Work out the finished part from the listing and answer in its coordinate system (mm). Face numbers are marked on the shaded views. A direction names the side the tool comes from. Round coordinates to 2 decimals unless told otherwise and drop trailing zeros. Order: outer loops, then holes, each group sorted by start corner. A loop starts at its lowest first (then second) coordinate and runs counter-clockwise, first axis right, second up. Notation, with made-up numbers: (31, 46) -> (40, 46) arc R13 ccw to (40, 53) -> close; hole circle Ø7 at (7, -9). An arc over 180 degrees is marked (long way). Use a Markdown table: item, result. Add a question column.
Item 1: A cutting plane is placed at D-D, the plane z = 23. Determine the outline of the cut face in (x, y), plus the area to 3 significant figures.
Item 2: Find the intervals of material crossed by L1, parallel to Z at x = 0, y = -13.25; L2, parallel to Z at x = 0, y = -18.35; L3, parallel to X at y = -17.5, z = -29, in increasing order. Write a range as [from, to].
Item 3: Flat-ended cylindrical pins translate along their axes: P1, Ø3, axis at x = 0.5, y = 2, coming from the -Z side; P2, Ø9.5, axis at x = 0, z = 23, coming from the +Y side; P3, Ø0.8, axis at x = 1, y = -17.5, coming from the -Z side; P4, Ø5.5, axis at x = 0, z = -7, coming from the -Y side. Find the tip coordinate at first contact, or state that the pin passes through.
Item 4: A cutting plane is placed at A-A, the plane z = -29.5. Determine the outline of the cut face in (x, y), plus the area to 3 significant figures.
Item 5: A tool of negligible diameter and unlimited length cuts with its end or side. For the marked faces 1, 2 and 3, from which of +Z, -Z, +X, -X, +Y, -Y can it reach the whole face along a straight path? Write none if from no direction.
Item 6: A cutting plane is placed at B-B, the plane z = -7. Determine the outline of the cut face in (x, y).
Item 7: For a pull along X with two mould halves and no side action, classify the marked faces 4, 5 and 6 as +X half, -X half, draft (parallel to the pull), parting line (faces both ways), or undercut.
Item 8: A cutting plane is placed at C-C, the plane y = -1.25. Determine the outline of the cut face in (x, z).
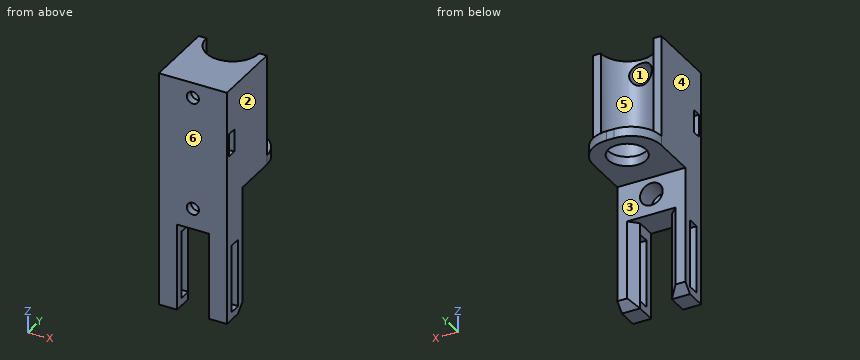
Autodesk Inventor part; units mm, degrees
ref_plane "YZ Plane" through (0, 0, 0) normal (1, 0, 0) x (0, 1, 0)
ref_plane "XZ Plane" through (0, 0, 0) normal (0, 1, 0) x (-1, 0, 0)
ref_plane "XY Plane" through (0, 0, 0) normal (0, 0, 1) x (1, 0, 0)
sketch "Sketch1" plane through (0, 0, 0) normal (0, 0, 1) x (1, 0, 0)
  circle A0 centre (0, 0) radius 7
  circle A1 centre (0, 0) radius 5
  circle A2 centre (0, 0) radius 1
  line L0 (-9, 0) -> (9, 0)
  line L1 (9, 0) -> (9, -19)
  line L2 (9, -19) -> (-9, -19)
  line L3 (-9, -19) -> (-9, 0)
  dimension "d11" = 14
  dimension "d12" = 10
  dimension "d13" = 2
  dimension "d18" = 19
  dimension "d19" = 18
extrude "Extrusion1" add sketch "Sketch1" along normal blind 27 contours L0 L1 L2 L3 A0 | A0 L0 A1 | A1 L0 A2 | A2 L0 picked at (6.2655, -0.5584) picked at (3.6182, -0.3989) picked at (-0.2952, -0.1549)
sketch "Sketch3" plane through (0, 0, 0) normal (0, 0, -1) x (-1, 0, 0)
  line L0 (9, -19) -> (9, 0)
  line L1 (-9, -19) -> (9, -19)
  line L2 (9, -19) -> (9, 8)
  line L3 (9, 8) -> (-9, 8)
  line L4 (-9, 8) -> (-9, -19)
  dimension "d22" = 27
extrude "Extrusion6" add sketch "Sketch3" along normal blind 2.5
extrude "Extrusion5" cut sketch "Sketch1" along normal blind 30 contours L0 A1 A0 | A0 L0 A1 | L0 A2 A1 | A1 L0 A2 | L0 A2 | A2 L0
extrude "Extrusion7" cut sketch "Sketch1" against normal through all contours L0 A2 A1 | A1 L0 A2 | L0 A2 | A2 L0
fillet "Fillet1" radius 8 2 edges at (-9, 8, -1.25) (9, 8, -1.25)
sketch "Sketch4" plane through (9, -19, 27) normal (1, 0, 0) x (0, 0, -1)
  line L0 (0, 0) -> (29.5, 0)
  line L1 (11.75, 3.5) -> (17.75, 3.5)
  line L2 (17.75, 3.5) -> (17.75, 1)
  line L3 (17.75, 1) -> (11.75, 1)
  line L4 (11.75, 1) -> (11.75, 3.5)
  point P0 (14.75, 0)
  point P1 (14.75, 1)
  dimension "d32" = 6
  dimension "d33" = 2.5
  dimension "d34" = 1
extrude "Extrusion8" cut sketch "Sketch4" against normal through all
sketch "Sketch5" plane through (0, 0, -2.5) normal (0, 0, -1) x (-1, 0, 0)
  line L0 (9, -19) -> (9, 0)
  line L1 (-9, -19) -> (9, -19)
  line L2 (9, -19) -> (9, -11.5)
  line L3 (9, -11.5) -> (-9, -11.5)
  line L4 (-9, -11.5) -> (-9, -19)
  dimension "d37" = 7.5
extrude "Extrusion9" add sketch "Sketch5" along normal blind 33
sketch "Sketch6" plane through (-9, -11.5, -2.5) normal (0, 1, 0) x (1, 0, 0)
  line L0 (4.8, 10) -> (13.2, 10)
  line L1 (13.2, 10) -> (13.2, 33)
  line L2 (13.2, 33) -> (4.8, 33)
  line L3 (4.8, 33) -> (4.8, 10)
  line L4 (0, 33) -> (18, 33)
  point P0 (9, -2.5)
  point P1 (9, 33)
  point P2 (9, 33)
  dimension "d45" = 23
  dimension "d47" = 0
  dimension "d69" = 8.4
extrude "Extrusion10" cut sketch "Sketch6" against normal blind 30
sketch "Sketch7" plane through (9, -19, 27) normal (1, 0, 0) x (0, 0, -1)
  line L0 (42.5, 5.35) -> (60.5, 5.35)
  line L1 (60.5, 5.35) -> (60.5, 2.15)
  line L2 (60.5, 2.15) -> (42.5, 2.15)
  line L3 (42.5, 2.15) -> (42.5, 5.35)
  line L4 (62.5, 7.5) -> (62.5, 0)
  line L5 (62.5, 7.5) -> (39.5, 7.5)
  point P0 (27, 19)
  point P1 (60.5, 3.75)
  point P2 (62.5, 3.75)
  point P3 (51.5, 5.35)
  point P4 (51, 7.5)
  point P5 (59.5, 7.5)
  dimension "d49" = 3.2
  dimension "d55" = 18
  dimension "d70" = 20
extrude "Extrusion11" cut sketch "Sketch7" against normal through all
sketch "Sketch8" plane through (-9, -11.5, -2.5) normal (0, 1, 0) x (1, 0, 0)
  circle A0 centre (9, 4.5) radius 3
  circle A1 centre (9, -25.5) radius 3
  line L0 (16, -29.5) -> (2, -29.5)
  point P0 (9, -2.5)
  dimension "d56" = 6
  dimension "d57" = 6
  dimension "d58" = 4
  dimension "d59" = 34
extrude "Extrusion12" cut sketch "Sketch8" along normal mid plane 11
sketch "Sketch9" plane through (0, -17, -7) normal (0, 1, 0) x (1, 0, 0)
  circle A0 centre (0, 0) radius 3
  circle A1 centre (0, 0) radius 1.6
  circle A2 centre (0, -30) radius 1.6
  point P0 (0, -7)
  dimension "d62" = 3.2
  dimension "d63" = 3.2
extrude "Extrusion13" cut sketch "Sketch9" against normal through all contours A1 | A2
chamfer "Chamfer2" distance 2.2 angle 45 4 edges at (4.2, -11.5, -24) (-4.2, -11.5, -24) (6.6, -11.5, -35.5) (-6.6, -11.5, -35.5)
properties part number "Solinoid holder v5"
Reported:
| question | item | result |
|---|---|---|
| 1 | outline | (-9, -19) -> (-1.6, -19) -> (-1.6, -17) -> (-3, -17) -> (-3, -6.32) arc R7 cw to (-7, 0) -> (-9, 0) -> close; (1.6, -19) -> (9, -19) -> (9, 0) -> (7, 0) arc R7 cw to (3, -6.32) -> (3, -17) -> (1.6, -17) -> close |
| 1 | area | 197 mm² |
| 2 | L1 | [-12.5, -10], [-4, 20], [26, 27] |
| 2 | L2 | [-12.5, -8.6], [-5.4, 21.4], [24.6, 27] |
| 2 | L3 | [-9, -4.2], [4.2, 9] |
| 3 | P1 | through |
| 3 | P2 | y = -5.14 |
| 3 | P3 | z = -12.5 |
| 3 | P4 | y = -19 |
| 4 | outline | (-9, -19) -> (-4.2, -19) -> (-4.2, -16.85) -> (-9, -16.85) -> close; (-9, -13.65) -> (-4.25, -13.65) -> (-6.4, -11.5) -> (-9, -11.5) -> close; (4.2, -19) -> (9, -19) -> (9, -16.85) -> (4.2, -16.85) -> close; (4.25, -13.65) -> (9, -13.65) -> (9, -11.5) -> (6.4, -11.5) -> close |
| 4 | area | 36.4 mm² |
| 5 | face 1 | +Y |
| 5 | face 2 | +Z, -Z, +X, +Y, -Y |
| 5 | face 3 | -Z, +X, -X, +Y |
| 6 | outline | (-9, -19) -> (-1.6, -19) -> (-1.6, -17) -> (-3, -17) -> (-3, -11.5) -> (-9, -11.5) -> close; (1.6, -19) -> (9, -19) -> (9, -11.5) -> (3, -11.5) -> (3, -17) -> (1.6, -17) -> close |
| 7 | face 4 | -X half |
| 7 | face 5 | undercut |
| 7 | face 6 | draft |
| 8 | outline | (-9, -2.5) -> (-4.84, -2.5) -> (-4.84, 0) -> (-6.89, 0) -> (-6.89, 27) -> (-9, 27) -> close; (4.84, -2.5) -> (9, -2.5) -> (9, 27) -> (6.89, 27) -> (6.89, 0) -> (4.84, 0) -> close |
